```python
from build123d import *

# Parameters (mm, degrees)
SKETCH_1_W               = 100
SKETCH_1_H               = 34.1
SKETCH_1_W_2             = 20
SKETCH_1_H_2             = 20
EXTRUDE_1_DEPTH          = 100
CUT_EXTRUDE_1_DEPTH      = 228.303332576
CUT_EXTRUDE_1_DEPTH_BACK = 228.303332576
SKETCH_2_W               = 70
SKETCH_2_H               = 15
CUT_EXTRUDE_2_DEPTH      = 221.148063812
CUT_EXTRUDE_2_DEPTH_BACK = 221.148063812
SKETCH_3_R               = 20
CUT_EXTRUDE_3_DEPTH      = 221.148063812
CUT_EXTRUDE_3_DEPTH_BACK = 221.148063812
SKETCH_4_R               = 10
FILLET_3_R               = 20
SKETCH_5_R               = 20
EXTRUDE_2_DEPTH          = 10
CUT_EXTRUDE_4_DEPTH      = 238.040629429
CUT_EXTRUDE_4_DEPTH_BACK = 238.040629429
SKETCH_6_R               = 15


with BuildPart() as part:
    # Эскиз1 → Бобышка-Вытянуть1 (new body)
    with BuildSketch(Plane.XY):
        with Locations((50, 17.05)):
            Rectangle(SKETCH_1_W, SKETCH_1_H)
        with BuildLine():
            Line((100, 34.1), (100, 0))
            Line((100, 0), (164.9, 0))
            Line((164.9, 0), (184.9, 0))
            Line((184.9, 0), (184.9, 34.1))
            Line((184.9, 34.1), (154.142135624, 34.1))
            ThreePointArc((154.142135624, 34.1), (140, 24.1), (125.857864376, 34.1))
            Line((125.857864376, 34.1), (100, 34.1))
        make_face()
        with BuildLine():
            Line((184.9, 50), (135.4, 99.5))
            Line((135.4, 99.5), (135.4, 53.377254638))
            ThreePointArc((135.4, 53.377254638), (148.831760866, 51.224355653), (155, 39.1))
            ThreePointArc((155, 39.1), (154.783978395, 36.563470319), (154.142135624, 34.1))
            Line((154.142135624, 34.1), (184.9, 34.1))
            Line((184.9, 34.1), (184.9, 50))
        make_face()
        with BuildLine():
            Line((100, 64.1), (100, 34.1))
            Line((100, 34.1), (125.857864376, 34.1))
            ThreePointArc((125.857864376, 34.1), (126.556784294, 45.754318257), (135.4, 53.377254638))
            Line((135.4, 53.377254638), (135.4, 99.5))
            Line((135.4, 99.5), (100, 64.1))
        make_face()
        with Locations((174.9, -10)):
            Rectangle(SKETCH_1_W_2, SKETCH_1_H_2)
    extrude(amount=EXTRUDE_1_DEPTH)

    # Эскиз2 → Вырез-Вытянуть1 (cut, two sides: drawn at the far end of the back side and taken through both)
    with BuildSketch(Plane(origin=(17.95, -17.95, 0), x_dir=(0, 0, 1), z_dir=(-0.7071067811865517, 0.7071067811865434, 0)).offset(-CUT_EXTRUDE_1_DEPTH_BACK)):
        with Locations((50, 158.599382901)):
            Rectangle(SKETCH_2_W, SKETCH_2_H)
    extrude(amount=CUT_EXTRUDE_1_DEPTH + CUT_EXTRUDE_1_DEPTH_BACK, mode=Mode.SUBTRACT)

    # Эскиз3 → Вырез-Вытянуть2 (cut, two sides: drawn at the far end of the back side and taken through both)
    with BuildSketch(Plane(origin=(0, 34.1, 0), x_dir=(1, 0, 0), z_dir=(0, 1, 0)).offset(-CUT_EXTRUDE_2_DEPTH_BACK)):
        with Locations((60, 0)):
            Circle(SKETCH_3_R)
        with Locations((60, -100)):
            Circle(SKETCH_3_R)
    extrude(amount=CUT_EXTRUDE_2_DEPTH + CUT_EXTRUDE_2_DEPTH_BACK, mode=Mode.SUBTRACT)

    # Эскиз4 → Вырез-Вытянуть3 (cut, two sides: drawn at the far end of the back side and taken through both)
    with BuildSketch(Plane(origin=(0, 34.1, 0), x_dir=(1, 0, 0), z_dir=(0, 1, 0)).offset(-CUT_EXTRUDE_3_DEPTH_BACK)):
        with BuildLine():
            Line((30, -80), (30, -20))
            ThreePointArc((30, -20), (20, -30), (10, -20))
            Line((10, -20), (10, -80))
            ThreePointArc((10, -80), (20, -70), (30, -80))
        make_face()
        with Locations((20, -20)):
            Circle(SKETCH_4_R)
        with Locations((20, -80)):
            Circle(SKETCH_4_R)
    extrude(amount=CUT_EXTRUDE_3_DEPTH + CUT_EXTRUDE_3_DEPTH_BACK, mode=Mode.SUBTRACT)

    # Скругление3
    fillet_3_edges = [part.edges().sort_by_distance(p)[0] for p in [
        (0, 17.05, 0),
        (0, 17.05, 100),
    ]]
    fillet(fillet_3_edges, radius=FILLET_3_R)

    # Эскиз5 → Бобышка-Вытянуть2 (add)
    with BuildSketch(Plane.XY.offset(100)):
        with Locations((140, 39.1)):
            Circle(SKETCH_5_R)
    extrude(amount=EXTRUDE_2_DEPTH)

    # Эскиз6 → Вырез-Вытянуть4 (cut, two sides: drawn at the far end of the back side and taken through both)
    with BuildSketch(Plane.XY.offset(110).offset(-CUT_EXTRUDE_4_DEPTH_BACK)):
        with Locations((140, 39.1)):
            Circle(SKETCH_6_R)
    extrude(amount=CUT_EXTRUDE_4_DEPTH + CUT_EXTRUDE_4_DEPTH_BACK, mode=Mode.SUBTRACT)


solid = part.part
```
Design review of the part built by this model. Coordinates are the model's own, in mm. A direction names the side the tool comes from. Coordinates: 2 decimals unless noted, no trailing zeros. Order: outer loops, then holes, each group sorted by start corner. A loop starts at its lowest first (then second) coordinate and runs counter-clockwise, first axis right, second up. Notation, with made-up numbers: (34, 58) -> (51, 58) arc R16 cw to (51, 73) -> close; hole circle Ø3 at (14, 56.5). An arc over 180 degrees is marked (long way). One line per item, written item: value. Start each with the question number.
Q1. For probe 1 along X at (y, z) = (21, 12.5); probe 2 along X at (y, z) = (12, 50.5); probe 3 along X at (y, z) = (39.1, 86.5), list the stretches that pass through material, from the lowest coordinate up.
Q2. Take a section at A-A, the plane z = 26.5. State the section outline as (x, y) points.
Q3. Insertion check: pin 1 Ø6 at (y, z) = (-9, 41.5) entering from -X; pin 2 Ø4 at (x, y) = (21, 30) entering from +Z; pin 3 Ø1.5 at (y, z) = (37, 44.5) entering from -X. Each pin has a flat end and moves straight along its axis. Give the tip position at first contact, or say it passes through.
Q4. Mouldability with a two-part tool opening along X and no side actions: class faces 3 (the flat face through (143, 54, 110)), 4 (the cylindrical face through (20, 17, 90)), 5 (the flat face through (0, 17, 50)) as pulls with the +X half, pulls with the -X half, needs draft (parallel to the pull), parting line crosses it, or undercut.
Q5. Take a section at D-D, the plane y = 76.5. State the section outline as (x, z) points.
Q6. Tool access review of faces 1 (the flat face through (10, 17, 50)), 2 (the flat face through (120, 27, 100)): name each direction out of +Z, -Z, +X, -X, +Y, -Y from which nothing blocks a thin tool from reaching the whole face with its end or side.
Values follow:
1. probe 1: x = 1.46 to 13.39, 26.61 to 44.39, 75.61 to 184.9
1. probe 2: x = 0 to 10, 30 to 184.9
1. probe 3: x = 100 to 125, 155 to 184.9
2. outline: (0, 0) -> (10, 0) -> (10, 34.1) -> (0, 34.1) -> close; (30, 0) -> (164.9, 0) -> (164.9, -20) -> (184.9, -20) -> (184.9, 28.79) -> (124.79, 88.89) -> (100, 64.1) -> (100, 34.1) -> (30, 34.1) -> close; hole circle Ø30 at (140, 39.1)
3. pin 1: stops at x = 164.9
3. pin 2: stops at z = 100
3. pin 3: stops at x = 100
4. face 3: needs draft
4. face 4: undercut
4. face 5: pulls with the -X half
5. outline: (112.4, 0) -> (158.4, 0) -> (158.4, 15) -> (137.19, 15) -> (137.19, 85) -> (158.4, 85) -> (158.4, 100) -> (112.4, 100) -> close
6. face 1: +Y, -Y
6. face 2: +Z
